The model under review builds one solid part; all positions refer to its coordinate system, in mm. A direction names the side the tool comes from. Round coordinates to 2 decimals unless told otherwise and drop trailing zeros. Order: outer loops, then holes, each group sorted by start corner. A loop starts at its lowest first (then second) coordinate and runs counter-clockwise, first axis right, second up.
1) Clearance check with a flat-ended pin moving along its axis: P1, Ø4, axis at x = -21, y = -33.5, coming from the -Z side. State where the tip first meets the part, or that it passes through.
2) Mouldability with a two-part tool opening along X and no side actions: class faces 1 (the face through (-17.4, -31, 9)), 2 (the face through (-24.1, -36.57, 11.21)), 3 (the face through (-24, -28, 11)) as pulls with the +X half, pulls with the -X half, needs draft (parallel to the pull), parting line crosses it, or undercut.
3) To check wall thickness, follow L1, parallel to X at y = -29.5, z = 7.5; L2, parallel to X at y = -34.25, z = 10.5; L3, parallel to Z at x = -20.5, y = -34. State the ranges of each line that lie inside material, in increasing order.
4) Consider section D-D (z = 9). Give the boundary of the cut face in (x, y), then the cut area to 3 significant figures.
5) Consider section B-B (x = -27). Give the boundary of the cut face in (y, z), then the cut area to 3 significant figures.
6) Machinability: for faces 4 (the face through (-21.15, -34, 11)), 5 (the face through (-23.44, -31.56, 10.4)), 6 (the face through (-25.8, -30, 8)), 7 (the face through (-26, -37, 11)), which of the approach directions +Z, -Z, +X, -X, +Y, -Y give a long, thin tool a straight path to every point of the face, cutting with its end or side? Answer none if there is none.
7) Consider section C-C (z = 11.25). Give the boundary of the cut face in (x, y).
8) Consider section A-A (z = 5.5). Give the boundary of the cut face in (x, y), then the cut area to 3 significant figures.
from build123d import *

# Parameters (mm, degrees)
PAD008_DEPTH            = 1.6
PAD009_DEPTH            = 1.6
LINEARPATTERN003_COUNT  = 2
LINEARPATTERN003_PITCH  = 8.4
FILLET012_R             = 1
FILLET013_R             = 1
FILLET014_R             = 1
FILLET015_R             = 1.5
BODY004_PLACEMENT_ANGLE = 90


with BuildPart() as part:
    # Sketch010 → Pad008 (new body)
    with BuildSketch(Plane.XY):
        with BuildLine():
            Line((-4.5, 5), (4.5, 5))
            Line((4.5, 5), (4.5, 1.25))
            Line((0, 1.25), (4.5, 1.25))
            ThreePointArc((0, 1.25), (-1.25, 0), (0, -1.25))
            Line((4.5, -1.25), (0, -1.25))
            Line((4.5, -1.25), (4.5, -5))
            Line((4.5, -5), (-4.5, -5))
            Line((-4.5, -5), (-4.5, 5))
        make_face()
    extrude(amount=PAD008_DEPTH)

    # Sketch011 (on DatumPlane) → Pad009 (join)
    with BuildSketch(Plane.XZ.offset(5)):
        Polygon((-4.5, 0), (-4.5, -5.6), (-2.5, -5.6), (-2.5, -4), (0.5, 0), align=None)
    pad009 = extrude(amount=-PAD009_DEPTH)

    # LinearPattern003: Pad009 ×2
    with Locations(*[(0, i * LINEARPATTERN003_PITCH, 0) for i in range(1, LINEARPATTERN003_COUNT)]):
        add(pad009)

    # Fillet012
    fillet012_edges = [part.edges().sort_by_distance(p)[0] for p in [
        (-2.5, -4.2, -5.6),
        (-2.5, 4.2, -5.6),
    ]]
    fillet(fillet012_edges, radius=FILLET012_R)

    # Fillet013
    fillet013_edges = [part.edges().sort_by_distance(p)[0] for p in [
        (-2.5, -4.2, -4),
        (-2.5, 4.2, -4),
    ]]
    fillet(fillet013_edges, radius=FILLET013_R)

    # Fillet014
    fillet014_edges = [part.edges().sort_by_distance(p)[0] for p in [
        (4.5, -5, 0.8),
        (4.5, 5, 0.8),
    ]]
    fillet(fillet014_edges, radius=FILLET014_R)

    # Fillet015
    fillet015_edges = [part.edges().sort_by_distance(p)[0] for p in [
        (4.5, -1.25, 0.8),
        (4.5, 1.25, 0.8),
    ]]
    fillet(fillet015_edges, radius=FILLET015_R)


with BuildPart() as part_1:
    # Body004 placement: moved
    add(part.part.moved(Location((-22.4, -32.5, 10.4))).rotate(Axis((-22.4, -32.5, 10.4), (0, 0, -1)), BODY004_PLACEMENT_ANGLE))


solid = part_1.part
Answer below:
1. P1: stops at z = 10.4
2. face 1: pulls with the +X half
2. face 2: undercut
2. face 3: needs draft
3. L1: x = -27.4 to -25.8, -19 to -17.4
3. L2: x = -27.4 to -23.65, -21.15 to -17.4
3. L3: z = 10.4 to 12
4. outline: (-27.4, -31.95) - (-25.8, -31.95) - (-25.8, -28) - (-27.4, -28) - close; (-19, -31.95) - (-17.4, -31.95) - (-17.4, -28) - (-19, -28) - close
4. area: 12.6 mm2
5. outline: (-36.8, 10.4) - (-33, 10.4) - (-30.2, 6.67) arc R1 cw to (-30, 6.07) - (-30, 5.8) arc R1 ccw to (-29, 4.8) - (-28, 4.8) - (-28, 12) - (-36.8, 12) - close
5. area: 31.1 mm2
6. face 4: +Z, -Z, -Y
6. face 5: -Z, -Y
6. face 6: -Z, +Y, -Y
6. face 7: +Z, -Z, +X, -X, -Y
7. outline: (-27.4, -36) arc R1 ccw to (-26.4, -37) - (-25.15, -37) arc R1.5 ccw to (-23.65, -35.5) - (-23.65, -32.5) arc R1.25 cw to (-21.15, -32.5) - (-21.15, -35.5) arc R1.5 ccw to (-19.65, -37) - (-18.4, -37) arc R1 ccw to (-17.4, -36) - (-17.4, -28) - (-27.4, -28) - close
8. outline: (-27.4, -29.95) - (-25.8, -29.95) - (-25.8, -28) - (-27.4, -28) - close; (-19, -29.95) - (-17.4, -29.95) - (-17.4, -28) - (-19, -28) - close
8. area: 6.25 mm2
